from build123d import *

# Parameters (mm, degrees)
SKETCH1_R             = 7.5
BOSS_EXTRUDE1_DEPTH   = 2
SKETCH2_R             = 9
BOSS_EXTRUDE2_DEPTH   = 0.9
SKETCH3_R             = 10
BOSS_EXTRUDE3_DEPTH   = 23
SKETCH5_R             = 2.1
CUT_EXTRUDE1_DEPTH    = 5.5
CUT_EXTRUDE2_DEPTH    = 20
SKETCH7_R             = 2.6
CUT_EXTRUDE3_DEPTH    = 30.509489999
CIRPATTERN1_START     = 3.039736726
CIRPATTERN1_OUTLINE_R = 2.6
CIRPATTERN1_DEPTH     = 6.960263374
CHAMFER1_SIZE         = 0.3


# Read off the part's stored shape, not the designer's step: CirPattern1
with BuildPart() as part:
    # Sketch1 → Boss-Extrude1 (new body)
    with BuildSketch(Plane(origin=(0, 0, 0), x_dir=(1, 0, 0), z_dir=(0, 1, 0))):
        with Locations(Location((0, 0, 0), (0, 0, 270))):
            Circle(SKETCH1_R)
    extrude(amount=BOSS_EXTRUDE1_DEPTH)

    # Sketch2 → Boss-Extrude2 (add)
    with BuildSketch(Plane(origin=(0, 2, 0), x_dir=(1, 0, 0), z_dir=(0, 1, 0))):
        with Locations(Location((0, 0, 0), (0, 0, 270))):
            Circle(SKETCH2_R)
    extrude(amount=BOSS_EXTRUDE2_DEPTH)

    # Sketch3 → Boss-Extrude3 (add)
    with BuildSketch(Plane(origin=(0, 2.9, 0), x_dir=(1, 0, 0), z_dir=(0, 1, 0))):
        with Locations(Location((0, 0, 0), (0, 0, 270))):
            Circle(SKETCH3_R)
    extrude(amount=BOSS_EXTRUDE3_DEPTH)

    # Sketch5 → Cut-Extrude1 (cut)
    with BuildSketch(Plane.XZ):
        with Locations(Location((4, 0, 0), (0, 0, 270))):
            Circle(SKETCH5_R)
        with Locations(Location((-2, -3.464101615, 0), (0, 0, 270))):
            Circle(SKETCH5_R)
        with Locations(Location((-2, 3.464101615, 0), (0, 0, 270))):
            Circle(SKETCH5_R)
    extrude(amount=-CUT_EXTRUDE1_DEPTH, mode=Mode.SUBTRACT)

    # Sketch6 → Cut-Extrude2 (cut)
    with BuildSketch(Plane(origin=(0, 25.9, 0), x_dir=(1, 0, 0), z_dir=(0, 1, 0))):
        with BuildLine():
            Line((-1.936491673, 3.5), (1.936491673, 3.5))
            ThreePointArc((1.936491673, 3.5), (0, -4), (-1.936491673, 3.5))
        make_face()
    extrude(amount=-CUT_EXTRUDE2_DEPTH, mode=Mode.SUBTRACT)

    # Sketch7 → Cut-Extrude3 (cut, through all)
    with BuildSketch(Plane.XY):
        with Locations(Location((0, 18.9, 0), (0, 0, 318.14230882))):
            Circle(SKETCH7_R)
    extrude(amount=-CUT_EXTRUDE3_DEPTH, mode=Mode.SUBTRACT)

    # CirPattern1 outline → CirPattern1 (cut)
    with BuildSketch(Plane(origin=(0, 0, 0), x_dir=(0.7071067811865509, 0, -0.707106781186544), z_dir=(0.707106781186544, 0, 0.707106781186551)).offset(CIRPATTERN1_START)):
        with Locations((0, 18.9)):
            Circle(CIRPATTERN1_OUTLINE_R)
    extrude(amount=CIRPATTERN1_DEPTH, mode=Mode.SUBTRACT)

    # Chamfer1
    chamfer1_edges = [part.edges().sort_by_distance(p)[0] for p in [
        (0, 0, -7.5),
    ]]
    chamfer(chamfer1_edges, length=CHAMFER1_SIZE)


solid = part.part
Verification items for the finished model (mm, model axes). A direction names the side the tool comes from. Give positions to 0.01 mm unless a question says otherwise; leave off trailing zeros. Order: outer loops, then holes, each group sorted by start corner. A loop starts at its lowest first (then second) coordinate and runs counter-clockwise, first axis right, second up. Notation, with made-up numbers: M 13,-39 L 19,-39 A36 ccw 19,-1 Z; hole C 61,76 d1. An arc over 180 degrees is marked long. Answer as a JSON object with one key per item and string values. Group by question number.
1) Mould release check, pull along X, two halves, no side actions. Record for faces 5 (the face through (0.33, 1.138, -7.493)), 6 (the face through (0.1, 25.9, 4.3)), 7 (the face through (-2, 5.5, 3)), 8 (the face through (-4.05, 2.71, 3.92)): released by +X, released by -X, zero draft, split by the parting line, or undercut.
2) Scan lines: line 1 along Y through (x, z) = (0, -7); line 2 along X through (y, z) = (3.2, 0); line 3 along Z through (x, y) = (0, 12.5). Record each from-to range of solid material in increasing order. Write a range as [from, to].
3) Access from +Z, -Z, +X, -X, +Y, -Y to the whole of each face (thin tool, end or side, straight path). Record for faces 1 (the face through (7.4, 2, -2)), 2 (the face through (0, 12, -3.5)), 3 (the face through (-3.83, 14.239, 9.237)), 4 (the face through (2.37, 17.83, -6.47)).
4) Cross-section at B-B (z = 0). Enter the section's corners in (x, y).
5) Cross-section at D-D (y = 5). Enter the section's corners in (x, z), then the cut area to 3 significant figures.
6) Cross-section at A-A (y = 18.9). Enter the section's corners in (x, z), then the cut area to 3 significant figures.
7) Depth check by flat-ended pin: pin 1 Ø1.5 at (y, z) = (4.5, -4.5) entering from +X; pin 2 Ø2 at (x, z) = (-2, 4.5) entering from -Y; pin 3 Ø2 at (y, z) = (13, 2.5) entering from +X. Enter the tip coordinate at first touch or a pass-through.
8) Cross-section at C-C (y = 9.75). Enter the section's corners in (x, z), then the cut area to 3 significant figures.
Result sheet:
{
 "1": {"face 5": "split by the parting line", "face 6": "zero draft", "face 7": "undercut", "face 8": "undercut"},
 "2": {"line 1": "y = [0, 16.3], [21.5, 25.9]", "line 2": "x = [-10, 1.9], [6.1, 10]", "line 3": "z = [-10, -3.5], [4, 10]"},
 "3": {"face 1": "-Y", "face 2": "+Y", "face 3": "+Y, -Y", "face 4": "-Z"},
 "4": {"outline": "M -10,2.9 L -9,2.9 L -9,2 L -7.5,2 L -7.5,0.3 L -7.2,0 L 1.9,0 L 1.9,5.5 L 6.1,5.5 L 6.1,0 L 7.2,0 L 7.5,0.3 L 7.5,2 L 9,2 L 9,2.9 L 10,2.9 L 10,25.9 L 4,25.9 L 4,5.9 L -4,5.9 L -4,25.9 L -10,25.9 Z"},
 "5": {"outline": "C 0,0 d20; hole C -2,-3.46 d4.2; hole C -2,3.46 d4.2; hole C 4,0 d4.2", "area": "273 mm2"},
 "6": {"outline": "M -2.6,-9.66 L -2.6,-3.04 A4 cw 0.31,3.99 L 4.99,8.67 A10 ccw long Z; M 2.6,-9.66 A10 ccw 8.67,4.99 L 3.99,0.31 A4 cw 2.6,-3.04 Z", "area": "200 mm2"},
 "7": {"pin 1": "stops at x = 9.27", "pin 2": "stops at y = 5.5", "pin 3": "stops at x = 9.89"},
 "8": {"outline": "C 0,0 d20; hole M -1.94,-3.5 L 1.94,-3.5 A4 ccw long Z", "area": "265 mm2"}
}
